Can you work these out from the model? Positions are in its coordinate system, mm. A direction names the side the tool comes from. Give positions to 0.01 mm unless a question says otherwise; leave off trailing zeros. Loops run counter-clockwise (first coordinate to the right, second up) from the corner with the lowest first, then second, coordinate; pieces in that order, holes last.
from build123d import *

# Parameters (mm, degrees)
F0_W     = 157.2524309158
F0_H     = 129.0383934975
F0_W_2   = 140.655875206
F0_H_2   = 115.3461933136
F1_DEPTH = 635
F2_R     = 5.08
F4_DEPTH = 157.2534309158


# Not quite as in the source:
# - a pattern or mirror of a feature is missing from the dataset's text; its kind, count and spacing are read off the source's solid


with BuildPart() as f1:
    # F0 (on Right) → F1 (new body, symmetric)
    with BuildSketch(Plane.YZ):
        Rectangle(F0_W, F0_H)
        Rectangle(F0_W_2, F0_H_2, mode=Mode.SUBTRACT)
    extrude(amount=F1_DEPTH, both=True)

    # F2
    f2_edges = [f1.edges().sort_by_distance(p)[0] for p in [
        (0, -78.626215, 64.519197),
        (0, -70.327938, 57.673097),
        (0, 70.327938, 57.673097),
        (0, 78.626215, 64.519197),
        (0, 78.626215, -64.519197),
        (0, 70.327938, -57.673097),
        (0, -70.327938, -57.673097),
        (0, -78.626215, -64.519197),
    ]]
    fillet(f2_edges, radius=F2_R)

    # F3 (on face) → F4 (cut, through all)
    with BuildSketch(Plane.XZ.offset(78.6262154579)):
        Polygon((635, -64.5191967487), (635, 64.5191967487), (505.9616065025, 64.5191967487), align=None)
    f4 = extrude(amount=-F4_DEPTH, mode=Mode.SUBTRACT)

    # F4_copies: F4 across plane
    add(f4.mirror(Plane(origin=(0, 0, 0), x_dir=(0, 0, -1), z_dir=(-1, 0, 0))), mode=Mode.SUBTRACT)


solid = f1.part
(1) Please list where these lines run through material, in increasing order: probe 1 along Y at (x, z) = (204.5, 9); probe 2 along Z at (x, y) = (-489, -44); probe 3 along Z at (x, y) = (-551, -4).
Returned:
probe 1: y = -78.63 to -70.33, 70.33 to 78.63
probe 2: z = -64.52 to -57.67, 57.67 to 64.52
probe 3: z = -64.52 to -57.67
(2) Suppose I cut it at D-D on x = 530. List the corners of the cut face in (y, z) for me, plus the area to 3 significant figures.
Returned:
outline: (-78.63, -59.44) arc R5.08 ccw to (-73.55, -64.52) - (73.55, -64.52) arc R5.08 ccw to (78.63, -59.44) - (78.63, 40.48) - (70.33, 40.48) - (70.33, -52.59) arc R5.08 cw to (65.25, -57.67) - (-65.25, -57.67) arc R5.08 cw to (-70.33, -52.59) - (-70.33, 40.48) - (-78.63, 40.48) - close
area: 2,710 mm2
(3) Thinking about a two-plate mould opening in Z: for faces 1 (the flat face through (9, -1, -57.673)), 2 (the flat face through (-570.18, -76.08, 0.3)), 3 (the flat face through (9, 78.626, -1)), which applies, pulls with the +Z half, pulls with the -Z half, needs draft (parallel to the pull), parting line crosses it, or undercut?
Returned:
face 1: undercut
face 2: pulls with the +Z half
face 3: needs draft
(4) Suppose I cut it at B-B on z = 25.5. List the corners of the cut face in (x, y) for me.
Returned:
outline: (-544.98, -78.63) - (544.98, -78.63) - (544.98, -70.33) - (-544.98, -70.33) - close; (-544.98, 70.33) - (544.98, 70.33) - (544.98, 78.63) - (-544.98, 78.63) - close
(5) Which directions (+Z, -Z, +X, -X, +Y, -Y) give clear straight access to the entire face, cutting with the end or side of a thin tool? Please do faces 4 (the flat face through (9, -1, -64.519)), 5 (the flat face through (9, -70.328, -1)).
Returned:
face 4: -Z, +X, -X, +Y, -Y
face 5: +X, -X
(6) Suppose I cut it at A-A on y = -46.5. List the corners of the cut face in (x, z) for me, plus the area to 3 significant figures.
Returned:
outline: (-635, -64.52) - (635, -64.52) - (628.15, -57.67) - (-628.15, -57.67) - close; (-512.81, 57.67) - (512.81, 57.67) - (505.96, 64.52) - (-505.96, 64.52) - close
area: 15,600 mm2
(7) Suppose I cut it at C-C on x = 30. List the corners of the cut face in (y, z) for me, plus the area to 3 significant figures.
Returned:
outline: (-78.63, -59.44) arc R5.08 ccw to (-73.55, -64.52) - (73.55, -64.52) arc R5.08 ccw to (78.63, -59.44) - (78.63, 59.44) arc R5.08 ccw to (73.55, 64.52) - (-73.55, 64.52) arc R5.08 ccw to (-78.63, 59.44) - close; hole (-70.33, -52.59) arc R5.08 ccw to (-65.25, -57.67) - (65.25, -57.67) arc R5.08 ccw to (70.33, -52.59) - (70.33, 52.59) arc R5.08 ccw to (65.25, 57.67) - (-65.25, 57.67) arc R5.08 ccw to (-70.33, 52.59) - close
area: 4,070 mm2
